```python
from build123d import *

# Parameters (mm, degrees)
SKETCH1_R           = 1.5
SKETCH1_W           = 5
SKETCH1_H           = 5
BOSS_EXTRUDE1_DEPTH = 5


with BuildPart() as part:
    # Sketch1 → Boss-Extrude1 (new body)
    with BuildSketch(Plane.XY):
        Polygon((0, 0), (0, 5.015390442), (-10, 5.015390442), (-10, 0), (-15, 0), (-15, 5.015390442), (-25, 5.015390442), (-25, 35.015390442), (15, 35.015390442), (15, 5.015390442), (5, 5.015390442), (5, 0), align=None)
        with Locations((-20, 20.015390442)):
            Circle(SKETCH1_R, mode=Mode.SUBTRACT)
        with Locations((10, 20.015390442)):
            Circle(SKETCH1_R, mode=Mode.SUBTRACT)
        with Locations((-20, 12.515390442)):
            Rectangle(SKETCH1_W, SKETCH1_H, mode=Mode.SUBTRACT)
        with Locations((-20, 27.515390442)):
            Rectangle(SKETCH1_W, SKETCH1_H, mode=Mode.SUBTRACT)
        with Locations((10, 12.515390442)):
            Rectangle(SKETCH1_W, SKETCH1_H, mode=Mode.SUBTRACT)
        with Locations((10, 27.515390442)):
            Rectangle(SKETCH1_W, SKETCH1_H, mode=Mode.SUBTRACT)
    extrude(amount=BOSS_EXTRUDE1_DEPTH)


solid = part.part
```
The model under review builds one solid part; all positions refer to its coordinate system, in mm. A direction names the side the tool comes from. Coordinates: 2 decimals unless noted, no trailing zeros. Loops run counter-clockwise (first coordinate to the right, second up) from the corner with the lowest first, then second, coordinate; pieces in that order, holes last. Notation, with made-up numbers: (-34.75, 53) -> (4.25, 53) arc R32 ccw to (4.25, 88) -> close; hole circle Ø4 at (48.25, 59). An arc over 180 degrees is marked (long way). Answer as CSV lines item,"result".
Item 1: Take a section at B-B, the plane x = 10. State the section outline as (y, z) points.
Results below:
outline,"(5.02, 0) -> (10.02, 0) -> (10.02, 5) -> (5.02, 5) -> close; (15.02, 0) -> (18.52, 0) -> (18.52, 5) -> (15.02, 5) -> close; (21.52, 0) -> (25.02, 0) -> (25.02, 5) -> (21.52, 5) -> close; (30.02, 0) -> (35.02, 0) -> (35.02, 5) -> (30.02, 5) -> close"
Item 2: Take a section at C-C, the plane y = 4. State the section outline as (x, z) points.
Results below:
outline,"(-15, 0) -> (-10, 0) -> (-10, 5) -> (-15, 5) -> close; (0, 0) -> (5, 0) -> (5, 5) -> (0, 5) -> close"
Item 3: For L1, parallel to X at y = 12.5, z = 4.2; L2, parallel to Y at x = -20, z = 2.6; L3, parallel to X at y = 20, z = 0.7, list the stretches that pass through material, from the lowest coordinate up.
Results below:
L1,"x = -25 to -22.5, -17.5 to 7.5, 12.5 to 15"
L2,"y = 5.02 to 10.02, 15.02 to 18.52, 21.52 to 25.02, 30.02 to 35.02"
L3,"x = -25 to -21.5, -18.5 to 8.5, 11.5 to 15"
Item 4: Take a section at D-D, the plane z = 1.8. Count the separate pieces of the cut face and the enclosed holes in it, and give its area (3 significant figures).
Results below:
separate pieces,"1"
enclosed holes,"6"
area,"1,140 mm2"
Item 5: Insertion check: pin 1 (2.5 mm diameter, centred on x = -21, z = 2, fed in from -Y). The pin has a flat end and moves straight along its axis. Give the tip position at first contact, or say it passes through.
Results below:
pin 1,"stops at y = 5.02"
Item 6: Take a section at A-A, the plane y = 27. State the section outline as (x, z) points, and give its area (3 significant figures).
Results below:
outline,"(-25, 0) -> (-22.5, 0) -> (-22.5, 5) -> (-25, 5) -> close; (-17.5, 0) -> (7.5, 0) -> (7.5, 5) -> (-17.5, 5) -> close; (12.5, 0) -> (15, 0) -> (15, 5) -> (12.5, 5) -> close"
area,"150 mm2"
Item 7: Machinability: for faces 1 (the flat face through (5, 3, 2)), 2 (the flat face through (-25, 20, 2)), 3 (the flat face through (10, 15.015, 2)), 4 (the flat face through (-20, 5.015, 2)), 5 (the flat face through (-10, 3, 2)), which of the approach directions +Z, -Z, +X, -X, +Y, -Y give a long, thin tool a straight path to every point of the face, cutting with its end or side? Answer none if there is none.
Results below:
face 1,"+Z, -Z, +X, -Y"
face 2,"+Z, -Z, -X, +Y, -Y"
face 3,"+Z, -Z"
face 4,"+Z, -Z, -X, -Y"
face 5,"+Z, -Z, -Y"
